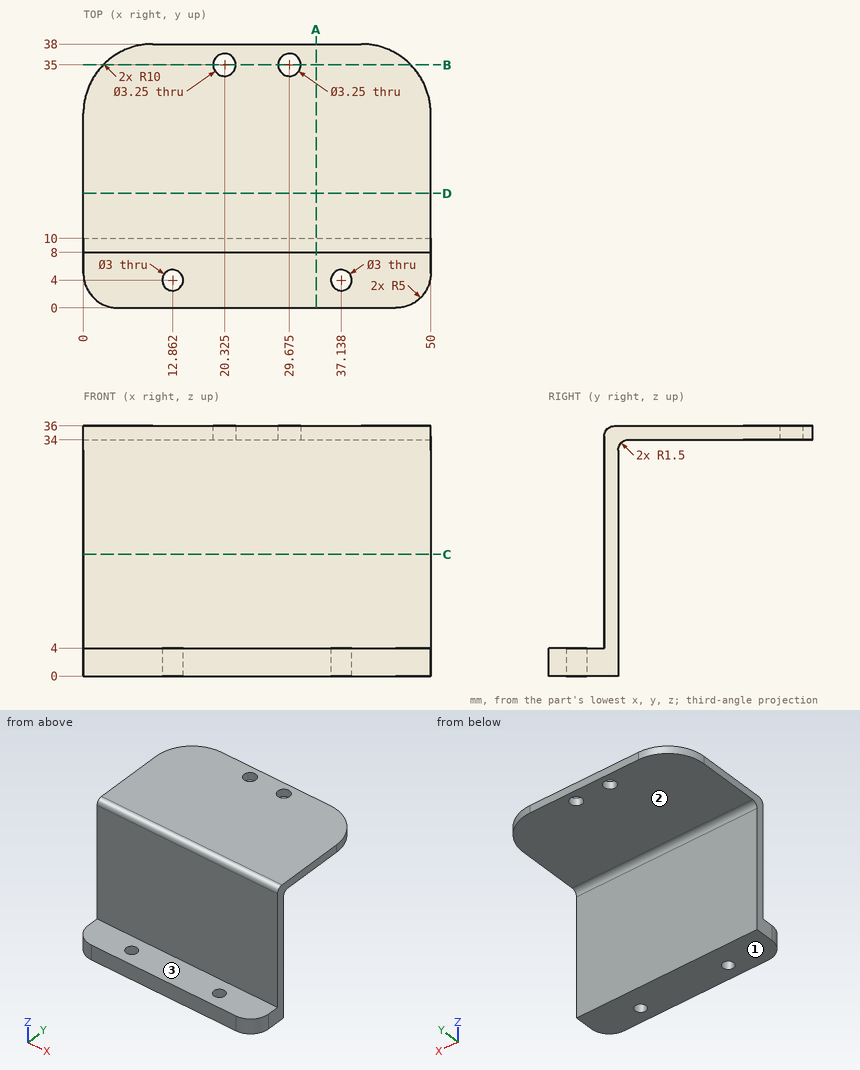
Can you work these out from the drawing? Everything is in mm from the part's minimum corner. A direction names the side the tool comes from. Round coordinates to 2 decimals unless told otherwise and drop trailing zeros. Loops run counter-clockwise (first coordinate to the right, second up) from the corner with the lowest first, then second, coordinate; pieces in that order, holes last. Notation, with made-up numbers: (-16.75, 71.25) - (11.25, 71.25) arc R26 cw to (11.25, 96.25) - close; hole circle Ø3 at (2, 36.25). An arc over 180 degrees is marked (long way). One line per question, with ' | ' between items. Start each with the question number.
Q1. Please list where these lines run through material, in increasing order: line 1 (Z direction, x = 40, y = 27.5); line 2 (Y direction, x = 27.5, z = 2.5); line 3 (Y direction, x = 41, z = 5.5). Write a range as [from, to].
Q2. I want a section at C-C (z = 17.5). Write out the boundary of the cut face in (x, y), then the cut area to 3 significant figures.
Q3. I want a section at D-D (y = 16.5). Write out the boundary of the cut face in (x, z), then the cut area to 3 significant figures.
Q4. For the marked faces 1, 2 and 3, which set-ups out of +Z, -Z, +X, -X, +Y, -Y let a thin tool reach every point of the face, with its end or its side?
Q5. I want a section at A-A (x = 33.5). Write out the boundary of the cut face in (y, z), then the cut area to 3 significant figures.
Q6. I want a section at B-B (y = 35). Write out the boundary of the cut face in (x, z).
Q7. Will these pins go through, and if not, where does the flat tip stop? pin 1 (10 mm diameter, centred on x = 33, z = 12, fed in from +Y); pin 2 (12 mm diameter, centred on x = 37.5, y = 30, fed in from -Z); pin 3 (10 mm diameter, centred on y = 11.5, z = 28, fed in from -X); pin 4 (3 mm diameter, centred on x = 8, z = 7.5, fed in from -Y).
Response values:
1) line 1: z = [34, 36] | line 2: y = [0, 10] | line 3: y = [8, 10]
2) outline: (0, 8) - (50, 8) - (50, 10) - (0, 10) - close | area: 100 mm²
3) outline: (0, 34) - (50, 34) - (50, 36) - (0, 36) - close | area: 100 mm²
4) face 1: -Z, +X, -X, +Y, -Y | face 2: -Z, +X, -X, +Y | face 3: +Z, +X, -X, -Y
5) outline: (0, 0) - (10, 0) - (10, 32.5) arc R1.5 cw to (11.5, 34) - (38, 34) - (38, 36) - (9.5, 36) arc R1.5 ccw to (8, 34.5) - (8, 4) - (0, 4) - close | area: 160 mm²
6) outline: (2.86, 34) - (18.7, 34) - (18.7, 36) - (2.86, 36) - close; (21.95, 34) - (28.05, 34) - (28.05, 36) - (21.95, 36) - close; (31.3, 34) - (47.14, 34) - (47.14, 36) - (31.3, 36) - close
7) pin 1: stops at y = 10 | pin 2: stops at z = 34 | pin 3: stops at x = 0 | pin 4: stops at y = 8
